The model under review builds one solid part; all positions refer to its coordinate system, in mm. A direction names the side the tool comes from. Round coordinates to 2 decimals unless told otherwise and drop trailing zeros. Write each loop counter-clockwise with the first axis right and the second up, starting at its lowest first coordinate (ties: lowest second). Pieces come first, ordered by that corner, then holes. Notation, with made-up numbers: (-25.5, -24.5) -> (21.5, -24.5) arc R11 ccw to (21.5, -4.5) -> close; hole circle Ø11 at (40.5, -20.75). An arc over 180 degrees is marked (long way). Answer as a JSON object with one key per item and string values. Group by question number.
1) Insertion check: pin 1 Ø10 at (x, y) = (8.5, 9) entering from -Z; pin 2 Ø4.5 at (x, y) = (-30, -10) entering from -Z; pin 3 Ø0.9 at (x, y) = (-12, -1.5) entering from +Z; pin 4 Ø1 at (y, z) = (12, 1) entering from +X. Each pin has a flat end and moves straight along its axis. Give the tip position at first contact, or say it passes through.
2) We need section A-A, the plane x = 20. Write out the cut boundary in (y, z).
3) Mouldability with a two-part tool opening along X and no side actions: class faces 1 (the flat face through (10, 28, 5)), 2 (the flat face through (-11, 45, 1)), 3 (the cylindrical face through (23, -16.5, 1)) as pulls with the +X half, pulls with the -X half, needs draft (parallel to the pull), parting line crosses it, or undercut.
4) We need section D-D, the plane z = 7.5. Write out the cut boundary in (x, y), then the cut area to 3 significant figures.
5) We need section C-C, the plane y = 20. Write out the cut boundary in (x, z), then the cut area to 3 significant figures.
6) Machinability: for faces 4 (the flat face through (39.64, -2, 3)), 5 (the flat face through (-8.77, 17.26, 7.6)), 6 (the flat face through (-10, 28, 5)), 7 (the flat face through (7.5, 23, 5)), which of the approach directions +Z, -Z, +X, -X, +Y, -Y give a long, thin tool a straight path to every point of the face, cutting with its end or side? Answer none if there is none.
7) To check wall thickness, follow probe 1 along Z at (x, y) = (8.35, 35); probe 2 along X at (y, z) = (13, 5.25); probe 3 along Y at (x, z) = (0, 0.9). State the ranges of each line that lie inside material, in increasing order. Write a range as [from, to].
8) We need section B-B, the plane y = -10. Write out the cut boundary in (x, z).
from build123d import *

# Parameters (mm, degrees)
PAD_DEPTH       = 2
PAD001_DEPTH    = 2.5
SKETCH002_R     = 1
SKETCH002_R_2   = 0.5
POCKET_DEPTH    = 5
SKETCH003_R     = 2.5
POCKET001_DEPTH = 2
SKETCH004_W     = 74.639832
SKETCH004_H     = 3
PAD002_DEPTH    = 3
SKETCH005_R     = 2.032906
POCKET002_DEPTH = 2


with BuildPart() as part:
    # Sketch → Pad (new body)
    with BuildSketch(Plane.XY):
        Polygon((-35, 0), (-15, 0), (-15, 45), (-10, 45), (-10, 0), (10, 0), (10, 45), (30, 45), (30, 0), (40, 0), (40, -20), (-35, -20), align=None)
    extrude(amount=PAD_DEPTH)

    # Sketch001 (on Face4 of Pad) → Pad001 (join)
    with BuildSketch(Plane.YZ.offset(-10)):
        Polygon((-3, 0), (-3, 2), (35, 12.5), (45, 2.20967), (45, 0), align=None)
    pad001 = extrude(amount=PAD001_DEPTH)

    # Sketch002 (on Face16 of Pad001) → Pocket (cut)
    with BuildSketch(Plane.YZ.offset(-7.5)):
        with Locations((35, 7.5)):
            Circle(SKETCH002_R)
        with Locations((35, 10)):
            Circle(SKETCH002_R_2)
        with Locations((35, 5)):
            Circle(SKETCH002_R_2)
    pocket = extrude(amount=-POCKET_DEPTH, mode=Mode.SUBTRACT)

    # Mirrored: Pad001, Pocket across YZ
    add(pad001.mirror(Plane.YZ))
    add(pocket.mirror(Plane.YZ), mode=Mode.SUBTRACT)

    # Sketch003 (on Face5 of Mirrored) → Pocket001 (cut)
    with BuildSketch(Plane.XY.offset(2)):
        with Locations((-30, -10)):
            Circle(SKETCH003_R)
        with Locations((-22.5, -15)):
            Circle(SKETCH003_R)
        with Locations((-12.5, -10)):
            Circle(SKETCH003_R)
        with Locations((35, -10)):
            Circle(SKETCH003_R)
        with Locations((25, -15)):
            Circle(SKETCH003_R)
        with Locations((12.5, -10)):
            Circle(SKETCH003_R)
        with Locations((0, -15)):
            Circle(SKETCH003_R)
    extrude(amount=-POCKET001_DEPTH, mode=Mode.SUBTRACT)

    # Sketch004 (on Face5 of Pocket001) → Pad002 (join)
    with BuildSketch(Plane.XY.offset(2)):
        with Locations((2.319916, -1.5)):
            Rectangle(SKETCH004_W, SKETCH004_H)
    extrude(amount=PAD002_DEPTH)

    # Sketch005 (on Face33 of Pad002) → Pocket002 (cut)
    with BuildSketch(Plane.XY.offset(2)):
        with Locations((20, 12)):
            Circle(SKETCH005_R)
    extrude(amount=-POCKET002_DEPTH, mode=Mode.SUBTRACT)


solid = part.part
Here are the results:
{
 "1": {"pin 1": "stops at z = 0", "pin 2": "passes through", "pin 3": "stops at z = 5", "pin 4": "stops at x = 30"},
 "2": {"outline": "(-20, 0) -> (9.97, 0) -> (9.97, 2) -> (0, 2) -> (0, 5) -> (-3, 5) -> (-3, 2) -> (-20, 2) -> close; (14.03, 0) -> (45, 0) -> (45, 2) -> (14.03, 2) -> close"},
 "3": {"face 1": "pulls with the +X half", "face 2": "needs draft", "face 3": "undercut"},
 "4": {"outline": "(-10, 16.9) -> (-7.5, 16.9) -> (-7.5, 34) -> (-10, 34) -> close; (-10, 36) -> (-7.5, 36) -> (-7.5, 39.86) -> (-10, 39.86) -> close; (7.5, 16.9) -> (10, 16.9) -> (10, 34) -> (7.5, 34) -> close; (7.5, 36) -> (10, 36) -> (10, 39.86) -> (7.5, 39.86) -> close", "area": "105 mm^2"},
 "5": {"outline": "(-15, 0) -> (-7.5, 0) -> (-7.5, 8.36) -> (-10, 8.36) -> (-10, 2) -> (-15, 2) -> close; (7.5, 0) -> (30, 0) -> (30, 2) -> (10, 2) -> (10, 8.36) -> (7.5, 8.36) -> close", "area": "91.8 mm^2"},
 "6": {"face 4": "+Z, +X, +Y, -Y", "face 5": "+Z, +X, -X", "face 6": "+Z, -X, +Y", "face 7": "+Z, -Z, +Y"},
 "7": {"probe 1": "z = [0, 4.5], [5.5, 6.5], [8.5, 9.5], [10.5, 12.5]", "probe 2": "x = [-10, -7.5], [7.5, 10]", "probe 3": "y = [-20, -17.5], [-12.5, 0]"},
 "8": {"outline": "(-35, 0) -> (-32.5, 0) -> (-32.5, 2) -> (-35, 2) -> close; (-27.5, 0) -> (-15, 0) -> (-15, 2) -> (-27.5, 2) -> close; (-10, 0) -> (10, 0) -> (10, 2) -> (-10, 2) -> close; (15, 0) -> (32.5, 0) -> (32.5, 2) -> (15, 2) -> close; (37.5, 0) -> (40, 0) -> (40, 2) -> (37.5, 2) -> close"}
}
